```python
from build123d import *

# Parameters (mm, degrees)
F0_W     = 200
F0_H     = 105
F1_DEPTH = 50
F2_T     = -2.5
F3_R     = 2.5
F3_R_2   = 5
F4_DEPTH = 105


with BuildPart() as f1:
    # F0 (on Top) → F1 (new body)
    with BuildSketch(Plane.XY):
        Rectangle(F0_W, F0_H)
    extrude(amount=F1_DEPTH)

    # F2
    f2_openings = [f1.faces().sort_by_distance(p)[0] for p in [
        (0, 0, 50),
    ]]
    offset(amount=F2_T, openings=f2_openings)

    # F3 (on face) → F4 (cut, through all)
    with BuildSketch(Plane.XZ.offset(52.5)):
        with Locations((-91, 46)):
            Circle(F3_R)
        with Locations((-78, 46)):
            Circle(F3_R)
        with Locations((-65, 46)):
            Circle(F3_R)
        with Locations((-52, 46)):
            Circle(F3_R)
        with Locations((-39, 46)):
            Circle(F3_R)
        with Locations((-26, 46)):
            Circle(F3_R)
        with Locations((-13, 46)):
            Circle(F3_R)
        with Locations((0, 46)):
            Circle(F3_R)
        with Locations((13, 46)):
            Circle(F3_R)
        with Locations((26, 46)):
            Circle(F3_R)
        with Locations((39, 46)):
            Circle(F3_R)
        with Locations((52, 46)):
            Circle(F3_R)
        with Locations((65, 46)):
            Circle(F3_R)
        with Locations((78, 46)):
            Circle(F3_R)
        with Locations((91, 46)):
            Circle(F3_R)
        with Locations((-39, 32)):
            Circle(F3_R)
        with Locations((0, 32)):
            Circle(F3_R)
        with Locations((39, 32)):
            Circle(F3_R)
        with Locations((-71.5, 22)):
            Circle(F3_R_2)
        with Locations((-19.5, 20)):
            Circle(F3_R)
        with Locations((58.5, 20)):
            Circle(F3_R)
        with Locations((85, 25)):
            Circle(F3_R)
    extrude(amount=-F4_DEPTH, mode=Mode.SUBTRACT)


solid = f1.part
```
Geometry: final body of the model. Coordinates: model frame, mm. A direction names the side the tool comes from. Coordinates: 2 decimals unless noted, no trailing zeros. Loops run counter-clockwise (first coordinate to the right, second up) from the corner with the lowest first, then second, coordinate; pieces in that order, holes last. Notation, with made-up numbers: M -26.5,33 L 31.5,33 A8 cw 31.5,44 Z; hole C 17.5,27.25 d9. An arc over 180 degrees is marked long. Put each result on its own line as item: value.
(1) Draft query along X for faces 1 (the face through (-1, 52.5, 25)), 2 (the face through (41.31, 51.23, 45.04)). Return one class per face: pulls with the +X half, pulls with the -X half, needs draft (parallel to the pull), parting line crosses it, or undercut.
Answer sheet:
face 1: needs draft
face 2: undercut
(2) Material intervals for probe 1 along X at (y, z) = (-29.5, 43); probe 2 along Y at (x, z) = (-34.5, 46); probe 3 along Z at (x, y) = (-13, 51.9), sorted ascending.
Answer sheet:
probe 1: x = -100 to -97.5, 97.5 to 100
probe 2: y = -52.5 to -50, 50 to 52.5
probe 3: z = 0 to 43.5, 48.5 to 50
(3) Cut plane A-A on x = 65. Return the cut outline in (y, z).
Answer sheet:
outline: M -52.5,0 L 52.5,0 L 52.5,43.5 L 50,43.5 L 50,2.5 L -50,2.5 L -50,43.5 L -52.5,43.5 Z; M -52.5,48.5 L -50,48.5 L -50,50 L -52.5,50 Z; M 50,48.5 L 52.5,48.5 L 52.5,50 L 50,50 Z
(4) Cut plane B-B on y = 44. Return the cut outline in (x, z).
Answer sheet:
outline: M -100,0 L 100,0 L 100,50 L 97.5,50 L 97.5,2.5 L -97.5,2.5 L -97.5,50 L -100,50 Z
(5) Access query for faces 3 (the face through (40.34, 51.23, 34.11)), 4 (the face through (-1, 1, 2.5)). Directions: +Z, -Z, +X, -X, +Y, -Y. A direction counts if a zero-diameter tool reaches every point of the face in a straight line with its end or side. Return the directions, or none.
Answer sheet:
face 3: +Y, -Y
face 4: +Z
(6) First-contact query: pin 1 (4 mm diameter, centred on x = -19.5, z = 20, fed in from +Y). Flat tip, straight axial feed; report the tip coordinate or a pass-through.
Answer sheet:
pin 1: passes through
(7) Cut plane C-C on x = 44. Return the cut outline in (y, z), then the cut area to 3 significant figures.
Answer sheet:
outline: M -52.5,0 L 52.5,0 L 52.5,50 L 50,50 L 50,2.5 L -50,2.5 L -50,50 L -52.5,50 Z
area: 500 mm^2
